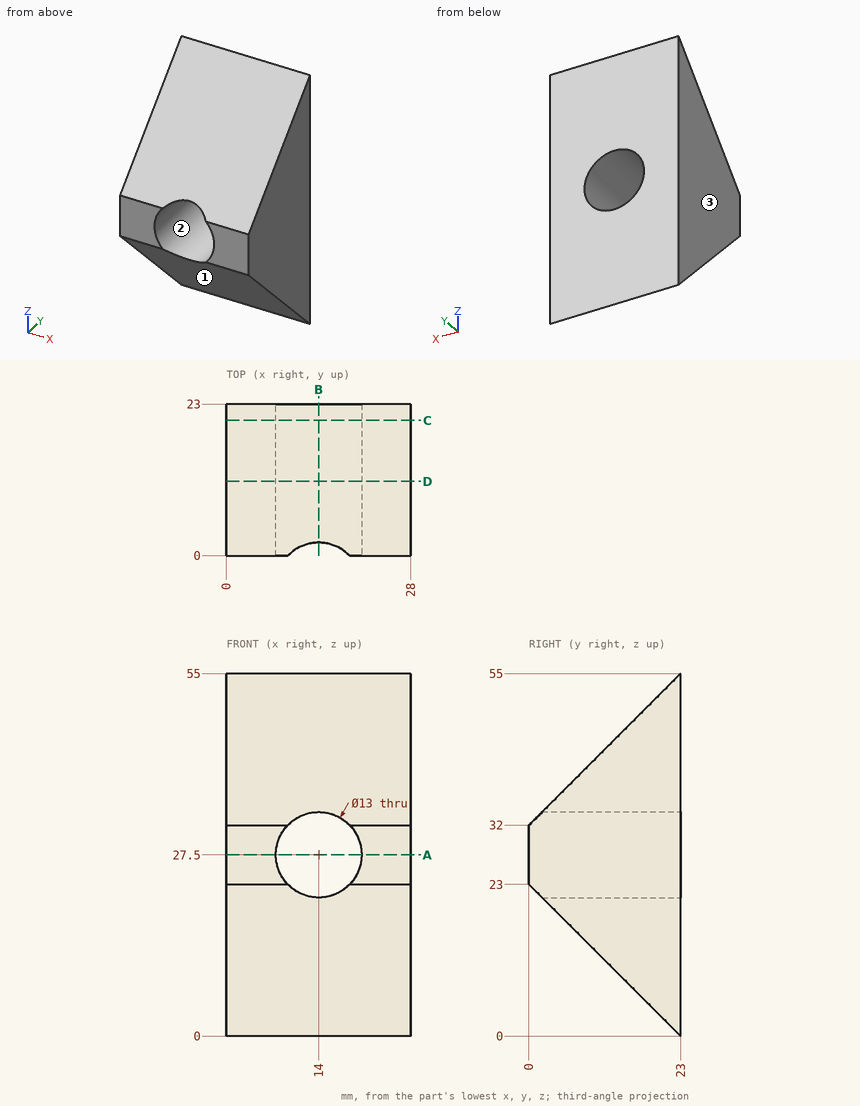
The drawing under review shows one solid part. Ordinate dimensions are in mm from its lowest x, y, z. Round coordinates to 2 decimals unless told otherwise and drop trailing zeros. Write each loop counter-clockwise with the first axis right and the second up, starting at its lowest first coordinate (ties: lowest second). Pieces come first, ordered by that corner, then holes. Notation, with made-up numbers: M 51,-39 L 109,-39 A31 ccw 109,-12 Z; hole C -25,-33 d2. An arc over 180 degrees is marked long. One line per item, written item: value. Start each with the question number.
(1) We need section B-B (x = 14). Give the boundary of the cut face in (y, z).
(2) The part is to be moulded in two halves that separate along X. For the marked faces 1, 2 and 3, say which applies: released by +X, released by -X, zero draft, split by the parting line, or undercut.
(3) We need section C-C (y = 20.5). Give the boundary of the cut face in (x, z), and give its area (3 significant figures).
(4) We need section D-D (y = 11.25). Give the boundary of the cut face in (x, z).
(5) Insertion check: pin 1 (1.5 mm diameter, centred on x = 4.5, y = 17.5, fed in from +Z); pin 2 (5 mm diameter, centred on x = 9, z = 9, fed in from -Y); pin 3 (3 mm diameter, centred on x = 8, y = 3.5, fed in from -Z). Each pin has a flat end and moves straight along its axis. Give the tip position at first contact, or say it passes through.
(6) We need section A-A (z = 27.5). Give the boundary of the cut face in (x, y).
(7) Wall thickness on line 1 (X direction, y = 5.25, z = 27.5); line 2 (Z direction, x = 14, y = 6.5); line 3 (Z direction, x = 11, y = 4): over which ranges is each line inside the solid? List them lowest first.
Result:
1. outline: M 2,21 L 23,0 L 23,21 Z; M 2,34 L 23,34 L 23,55 Z
2. face 1: zero draft
2. face 2: undercut
2. face 3: released by -X
3. outline: M 0,2.5 L 28,2.5 L 28,52.5 L 0,52.5 Z; hole C 14,27.5 d13
3. area: 1,270 mm²
4. outline: M 0,11.75 L 28,11.75 L 28,43.25 L 0,43.25 Z; hole C 14,27.5 d13
5. pin 1: z = 50.25
5. pin 2: y = 11.5
5. pin 3: z = 18
6. outline: M 0,0 L 7.5,0 L 7.5,23 L 0,23 Z; M 20.5,0 L 28,0 L 28,23 L 20.5,23 Z
7. line 1: 0 to 7.5, 20.5 to 28
7. line 2: 16.5 to 21, 34 to 38.5
7. line 3: 19 to 21.73, 33.27 to 36
